```python
from build123d import *

# Parameters (mm, degrees)
SKETCH_1_R           = 27
EXTRUDE_1_DEPTH      = 8
SKETCH_2_R           = 22.5
EXTRUDE_2_DEPTH      = 54
SKETCH_3_R           = 9
EXTRUDE_3_DEPTH      = 13
SKETCH_4_R           = 15
CUT_EXTRUDE_1_DEPTH  = 56
CUT_EXTRUDE_2_REACH  = 74.815
SKETCH_7_R           = 9
SKETCH_8_W           = 74
SKETCH_8_H           = 20
EXTRUDE_4_DEPTH      = 7
EXTRUDE_5_REACH      = 96.25
EXTRUDE_5_END_RADIUS = 22.5
SKETCH_9_W           = 28
SKETCH_9_H           = 20
CUT_EXTRUDE_3_REACH  = 62.614
SKETCH_10_W          = 22
SKETCH_10_H          = 6
EXTRUDE_7_REACH      = 104.259
EXTRUDE_7_END_RADIUS = 22.5
SKETCH_12_R          = 11
EXTRUDE_8_REACH      = 98.794
EXTRUDE_8_END_RADIUS = 22.5
SKETCH_15_R          = 11
SKETCH_13_R          = 7.5
CUT_EXTRUDE_6_DEPTH  = 56
SKETCH_16_R          = 7.5
EXTRUDE_9_DEPTH      = 13
SKETCH_17_R          = 4
CUT_EXTRUDE_7_DEPTH  = 30
SKETCH_18_R          = 3
CUT_EXTRUDE_8_DEPTH  = 30


with BuildPart() as part:
    # 草图1 → 凸台-拉伸1 (new body)
    with BuildSketch(Plane.XY):
        Circle(SKETCH_1_R)
    extrude(amount=-EXTRUDE_1_DEPTH)

    # 草图2 → 凸台-拉伸2 (add)
    with BuildSketch(Plane.XY):
        Circle(SKETCH_2_R)
    extrude(amount=EXTRUDE_2_DEPTH)

    # 草图3 → 凸台-拉伸3 (add)
    with BuildSketch(Plane.XY.offset(54)):
        Polygon((0, 10.011106999), (-13, 2.505553499), (-13, -12.505553499), (0, -20.011106999), (13, -12.505553499), (13, 2.505553499), align=None)
        with Locations(Location((0, -5, 0), (0, 0, 180))):
            Circle(SKETCH_3_R, mode=Mode.SUBTRACT)
    extrude(amount=EXTRUDE_3_DEPTH)

    # 草图4 → 切除-拉伸1 (cut)
    with BuildSketch(Plane(origin=(0, 0, -8), x_dir=(-1, 0, 0), z_dir=(0, 0, -1))):
        Circle(SKETCH_4_R)
    extrude(amount=-CUT_EXTRUDE_1_DEPTH, mode=Mode.SUBTRACT)

    # 草图7 → 切除-拉伸2 (cut, up to next)
    with BuildSketch(Plane.XY.offset(54), mode=Mode.PRIVATE) as cut_extrude_2_sk1:
        with Locations(Location((0, -5, 0), (0, 0, 180))):
            Circle(SKETCH_7_R)
    cut_extrude_2_tool1 = extrude(cut_extrude_2_sk1.sketch, amount=-CUT_EXTRUDE_2_REACH, mode=Mode.PRIVATE) & part.part
    add(cut_extrude_2_tool1.solids().sort_by_distance((0, -5, 54))[0], mode=Mode.SUBTRACT)

    # 草图8 → 凸台-拉伸4 (add)
    with BuildSketch(Plane(origin=(0, -28, 0), x_dir=(1, 0, 0), z_dir=(0, 1, 0))):
        with Locations((0, -18)):
            Rectangle(SKETCH_8_W, SKETCH_8_H)
    extrude(amount=EXTRUDE_4_DEPTH)

    # 凸台-拉伸5: up to this cylinder (the profile starts outside it)
    extrude_5_end = Plane(origin=(0, 0, 18), z_dir=(0, 0, -1)) * Cylinder(EXTRUDE_5_END_RADIUS, 238.5, mode=Mode.PRIVATE)
    # 草图9 → 凸台-拉伸5 (add, up to the surface)
    with BuildSketch(Plane.XZ.offset(28), mode=Mode.PRIVATE) as extrude_5_sk1:
        with Locations((0, 18)):
            Rectangle(SKETCH_9_W, SKETCH_9_H)
    extrude_5_tool1 = extrude(extrude_5_sk1.sketch, amount=-EXTRUDE_5_REACH, mode=Mode.PRIVATE) - extrude_5_end
    add(extrude_5_tool1.solids().sort_by_distance((0, -28, 18))[0])

    # 草图10 → 切除-拉伸3 (cut, up to next)
    with BuildSketch(Plane.XY.offset(28), mode=Mode.PRIVATE) as cut_extrude_3_sk1:
        with Locations((0, -28)):
            Rectangle(SKETCH_10_W, SKETCH_10_H)
    cut_extrude_3_tool1 = extrude(cut_extrude_3_sk1.sketch, amount=-CUT_EXTRUDE_3_REACH, mode=Mode.PRIVATE) & part.part
    add(cut_extrude_3_tool1.solids().sort_by_distance((0, -28, 28))[0], mode=Mode.SUBTRACT)

    # 凸台-拉伸7: up to this cylinder (the profile starts outside it)
    extrude_7_end = Plane(origin=(0, 0, 34), z_dir=(0, 0, -1)) * Cylinder(EXTRUDE_7_END_RADIUS, 254.518, mode=Mode.PRIVATE)
    # 草图12 → 凸台-拉伸7 (add, up to the surface)
    with BuildSketch(Plane(origin=(35, 0, 0), x_dir=(0, 0, -1), z_dir=(1, 0, 0)), mode=Mode.PRIVATE) as extrude_7_sk1:
        with Locations((-34, 5)):
            Circle(SKETCH_12_R)
    extrude_7_tool1 = extrude(extrude_7_sk1.sketch, amount=-EXTRUDE_7_REACH, mode=Mode.PRIVATE) - extrude_7_end
    add(extrude_7_tool1.solids().sort_by_distance((35, 5, 34))[0])

    # 凸台-拉伸8: up to this cylinder (the profile starts outside it)
    extrude_8_end = Plane(origin=(0, 0, 34), z_dir=(0, 0, -1)) * Cylinder(EXTRUDE_8_END_RADIUS, 243.588, mode=Mode.PRIVATE)
    # 草图15 → 凸台-拉伸8 (add, up to the surface)
    with BuildSketch(Plane(origin=(-27, 0, 0), x_dir=(0, 0, -1), z_dir=(1, 0, 0)), mode=Mode.PRIVATE) as extrude_8_sk1:
        with Locations((-34, 5)):
            Circle(SKETCH_15_R)
    extrude_8_tool1 = extrude(extrude_8_sk1.sketch, amount=EXTRUDE_8_REACH, mode=Mode.PRIVATE) - extrude_8_end
    add(extrude_8_tool1.solids().sort_by_distance((-27, 5, 34))[0])

    # 草图13 → 切除-拉伸6 (cut)
    with BuildSketch(Plane(origin=(35, 0, 0), x_dir=(0, 0, -1), z_dir=(1, 0, 0))):
        with Locations((-34, 5)):
            Circle(SKETCH_13_R)
    extrude(amount=-CUT_EXTRUDE_6_DEPTH, mode=Mode.SUBTRACT)

    # 草图16 → 凸台-拉伸9 (add)
    with BuildSketch(Plane.ZY.offset(27)):
        with Locations(Location((34, 5, 0), (0, 0, 180))):
            Circle(SKETCH_16_R)
    extrude(amount=EXTRUDE_9_DEPTH)

    # 草图17 → 切除-拉伸7 (cut)
    with BuildSketch(Plane.ZY.offset(40)):
        with Locations((34, 5)):
            Circle(SKETCH_17_R)
    extrude(amount=-CUT_EXTRUDE_7_DEPTH, mode=Mode.SUBTRACT)

    # 草图18 → 切除-拉伸8 (cut)
    with BuildSketch(Plane(origin=(0, -21, 0), x_dir=(1, 0, 0), z_dir=(0, 1, 0))):
        with Locations(Location((-27, -18, 0), (0, 0, 270))):
            Circle(SKETCH_18_R)
        with Locations(Location((27, -18, 0), (0, 0, 270))):
            Circle(SKETCH_18_R)
    extrude(amount=-CUT_EXTRUDE_8_DEPTH, mode=Mode.SUBTRACT)


solid = part.part
```
Model file for the job. Use its own axes, mm. A direction names the side the tool comes from. Coordinates: 2 decimals unless noted, no trailing zeros. Loops run counter-clockwise (first coordinate to the right, second up) from the corner with the lowest first, then second, coordinate; pieces in that order, holes last. Notation, with made-up numbers: M -16.5,-4 L 18.5,-4 A18 ccw 18.5,24 Z; hole C 44,-38.5 d9. An arc over 180 degrees is marked long. Use CSV: the item, a comma, the result in double quotes. Start each with the question number.
1. Band-saw the part on D-D, the plane y = 8. Give the number of separate pieces and of enclosed holes in the cut face, then the cut area to 3 significant figures.
2. Band-saw the part on A-A, the plane z = 12.5. List the corners of the cut face in (x, y), then the cut area to 3 significant figures.
3. Two-plate mould, pull along Z, no slides. Class faces 1 (the cylindrical face through (24.8, 12.436, 34.976)), 2 (the flat face through (6.6, 6.2, 60.4)), 3 (the flat face through (12, -12, -8)), 4 (the cylindrical face through (27.675, 15.906, 35.432)): pulls with the +Z half, pulls with the -Z half, needs draft (parallel to the pull), parting line crosses it, or undercut.
4. Band-saw the part on B-B, the plane z = 34. List the corners of the cut face in (x, y).
5. Probe probe 1 along X at (y, z) = (-24, 18); probe 2 along Z at (x, y) = (23.75, 5); probe 3 along Y at (x, z) = (-25.75, 34). List the from-to ranges inside material, lowest first. Write a range as [from, to].
6. Band-saw the part on C-C, the plane y = -5. List the corners of the cut face in (x, z), then the cut area to 3 significant figures.
7. Flat gauge pins, fed straight in: pin 1 (3.5 mm diameter, centred on y = -18.5, z = 15, fed in from -X); pin 2 (2 mm diameter, centred on y = 10.5, z = 1.5, fed in from -X); pin 3 (5 mm diameter, centred on x = -27.5, y = -14.5, fed in from +Z) (1 decimal); pin 4 (10 mm diameter, centred on x = 1, z = 19, fed in from -Y). Where does each tip first touch, or does it go through?
8. Tool access for faces 5 (the cylindrical face through (-33.409, 4.67, 41.493)), 6 (the flat face through (0, -25, 18)), 7 (the flat face through (-21, 2, 31)), 8 (the cylindrical face through (-2.93, 22.31, 26.62)), 9 (the cylindrical face through (-6.92, -13.31, 19.61)): list every direction of +Z, -Z, +X, -X, +Y, -Y with a clear straight run to the whole face (end or side of a thin tool).
Entries:
1,separate pieces,"3"
1,enclosed holes,"0"
1,area,"1,430 mm2"
2,outline,"M -37,-28 L -11,-28 L -11,-25 L 11,-25 L 11,-28 L 37,-28 L 37,-21 L 14,-21 L 14,-17.61 A22.5 ccw long -14,-17.61 L -14,-21 L -37,-21 Z; hole C 0,0 d30"
2,area,"1,340 mm2"
3,face 1,"undercut"
3,face 2,"needs draft"
3,face 3,"pulls with the -Z half"
3,face 4,"undercut"
4,outline,"M -40,-2.5 L -27,-2.5 L -27,-6 L -21.69,-6 A22.5 ccw 21.69,-6 L 35,-6 L 35,-2.5 L 14.79,-2.5 A15 cw -14.79,-2.5 L -21,-2.5 L -21,1 L -40,1 Z; M -40,9 L -21,9 L -21,12.5 L -8.29,12.5 A15 cw 8.29,12.5 L 35,12.5 L 35,16 L 15.82,16 A22.5 ccw -15.82,16 L -27,16 L -27,12.5 L -40,12.5 Z"
5,probe 1,"x = [-37, -30], [-24, 24], [30, 37]"
5,probe 2,"z = [-8, 0], [23, 26.5], [41.5, 45]"
5,probe 3,"y = [-6, 1], [9, 16]"
6,outline,"M -27,29.42 L -21.94,29.42 L -21.94,0 L -26.53,0 L -26.53,-8 L -14.14,-8 L -14.14,48 L -9,48 L -9,67 L -13,67 L -13,54 L -21.94,54 L -21.94,38.58 L -27,38.58 Z; M 9,48 L 14.14,48 L 14.14,-8 L 26.53,-8 L 26.53,0 L 21.94,0 L 21.94,29.42 L 35,29.42 L 35,38.58 L 21.94,38.58 L 21.94,54 L 13,54 L 13,67 L 9,67 Z"
6,area,"1,370 mm2"
7,pin 1,"stops at x = -15.02"
7,pin 2,"stops at x = -20.4"
7,pin 3,"passes through"
7,pin 4,"stops at y = -25"
8,face 5,"-X"
8,face 6,"+Z, -Y"
8,face 7,"+X"
8,face 8,"none"
8,face 9,"-Z"
